from build123d import *

# Parameters (mm, degrees)
F0_W     = 158.75
F0_H     = 50.8
F0_R     = 6.35
F0_W_2   = 15.875
F1_DEPTH = 3.175
F0_H_2   = 3.175
F2_DEPTH = 85.725
F3_DEPTH = 120.65


with BuildPart() as f1:
    # F0 (on Front) → F1 (new body)
    with BuildSketch(Plane.XZ):
        with Locations((0, -50.8)):
            Rectangle(F0_W, F0_H)
        with Locations((0, 50.8)):
            Rectangle(F0_W, F0_H)
        Polygon((95.25, 25.4), (95.25, -25.4), (79.375, -25.4), (79.375, -76.2), (107.95, -76.2), (107.95, 76.2), (79.375, 76.2), (79.375, 25.4), align=None)
        with Locations((95.25, -57.15)):
            Circle(F0_R, mode=Mode.SUBTRACT)
        with Locations((95.25, 57.15)):
            Circle(F0_R, mode=Mode.SUBTRACT)
        Polygon((-79.375, -76.2), (-79.375, -25.4), (-95.25, -25.4), (-95.25, 25.4), (-79.375, 25.4), (-79.375, 76.2), (-107.95, 76.2), (-107.95, -76.2), align=None)
        with Locations((-95.25, -57.15)):
            Circle(F0_R, mode=Mode.SUBTRACT)
        with Locations((-95.25, 57.15)):
            Circle(F0_R, mode=Mode.SUBTRACT)
        Rectangle(F0_W, F0_H)
        with Locations((-87.3125, 0)):
            Rectangle(F0_W_2, F0_H)
        with Locations((87.3125, 0)):
            Rectangle(F0_W_2, F0_H)
    extrude(amount=F1_DEPTH)

    # F0 (on Front) → F2 (join)
    with BuildSketch(Plane.XZ):
        with Locations((0, -50.8)):
            Rectangle(F0_W, F0_H)
        Rectangle(F0_W, F0_H)
        with Locations((0, 50.8)):
            Rectangle(F0_W, F0_H)
        with Locations((0, 77.7875)):
            Rectangle(F0_W, F0_H_2)
        with Locations((0, -77.7875)):
            Rectangle(F0_W, F0_H_2)
    extrude(amount=-F2_DEPTH)

    # F0 (on Front) → F3 (join)
    with BuildSketch(Plane.XZ):
        with Locations((-87.3125, 0)):
            Rectangle(F0_W_2, F0_H)
        Rectangle(F0_W, F0_H)
        with Locations((87.3125, 0)):
            Rectangle(F0_W_2, F0_H)
    extrude(amount=F3_DEPTH)


solid = f1.part
Geometry: final body of the model. Coordinates: model frame, mm. A direction names the side the tool comes from. Coordinates: 2 decimals unless noted, no trailing zeros. Order: outer loops, then holes, each group sorted by start corner. A loop starts at its lowest first (then second) coordinate and runs counter-clockwise, first axis right, second up. Notation, with made-up numbers: (-11, 28.25) - (31, 28.25) arc R17 ccw to (31, 39.25) - close; hole circle Ø1 at (-32, 63). An arc over 180 degrees is marked (long way). Use one line per item in the form item = value.
1) Set-up query: faces 1 (the face through (79.375, 42, -1)), 2 (the face through (-95.25, -61, 0)), 3 (the face through (1, -61, 25.4)). Return all of +Z, -Z, +X, -X, +Y, -Y with unobstructed straight access to the full face (end or side cutting, diameter ignored); none if empty.
Solutions:
face_1 = +Z, -Z, +X, +Y
face_2 = +Z, -Z, -X, -Y
face_3 = +Z, +X, -X, -Y
2) Pin query (flat end, axial travel): pin 1 (5 mm diameter, centred on x = -19, y = -50, fed in from -Z); pin 2 (16.5 mm diameter, centred on x = -95.25, z = -57.15, fed in from -Y) (3 decimals); pin 3 (4 mm diameter, centred on x = 84.5, z = 14.5, fed in from +Y). Return the tip coordinate at first contact, or that it passes through.
Solutions:
pin_1 = -25.4
pin_2 = -3.175
pin_3 = 0
3) Ray query, L1, parallel to Z at x = 95.25, y = -1.15; L2, parallel to X at y = -1, z = 57; L3, parallel to Y at x = -68, z = -43.5 (3 decimals). Return the intervals inside material, ascending.
Solutions:
L1 = -76.2 to -63.5, -50.8 to 50.8, 63.5 to 76.2
L2 = -107.95 to -101.6, -88.9 to 88.9, 101.6 to 107.95
L3 = -3.175 to 85.725
4) Section C-C (z = 19). Return loops of the section in (x, y) (3 decimals).
Solutions:
outline = (-107.95, -3.175) - (-95.25, -3.175) - (-95.25, -120.65) - (95.25, -120.65) - (95.25, -3.175) - (107.95, -3.175) - (107.95, 0) - (79.375, 0) - (79.375, 85.725) - (-79.375, 85.725) - (-79.375, 0) - (-107.95, 0) - close
5) Mould query, pull axis X, two halves, no side actions, for faces 4 (the face through (-1, 85.725, 1)), 5 (the face through (101.307, -1.565, -55.243)), 6 (the face through (-79.375, 42, 1)). Classes: +X half, -X half, draft (parallel to the pull), parting line (faces both ways), or undercut.
Solutions:
face_4 = draft
face_5 = undercut
face_6 = -X half
6) Section A-A (z = 57.15). Return loops of the section in (x, y) (3 decimals).
Solutions:
outline = (-107.95, -3.175) - (-101.6, -3.175) - (-101.6, 0) - (-107.95, 0) - close; (-88.9, -3.175) - (88.9, -3.175) - (88.9, 0) - (79.375, 0) - (79.375, 85.725) - (-79.375, 85.725) - (-79.375, 0) - (-88.9, 0) - close; (101.6, -3.175) - (107.95, -3.175) - (107.95, 0) - (101.6, 0) - close
7) Section D-D (y = 41). Return loops of the section in (x, z) (3 decimals), then the cut area to 3 significant figures.
Solutions:
outline = (-79.375, -79.375) - (79.375, -79.375) - (79.375, 79.375) - (-79.375, 79.375) - close
area = 25,200 mm^2
8) Section B-B (x = -29.5). Return loops of the section in (y, z) (3 decimals), then the cut area to 3 significant figures.
Solutions:
outline = (-120.65, -25.4) - (-3.175, -25.4) - (-3.175, -76.2) - (0, -76.2) - (0, -79.375) - (85.725, -79.375) - (85.725, 79.375) - (0, 79.375) - (0, 76.2) - (-3.175, 76.2) - (-3.175, 25.4) - (-120.65, 25.4) - close
area = 20,100 mm^2
